Geometry check sheet. Reference: drawing and pictorial views, mm from the part's lowest x, y, z. Round coordinates to 2 decimals unless told otherwise and drop trailing zeros. Write each loop counter-clockwise with the first axis right and the second up, starting at its lowest first coordinate (ties: lowest second). Pieces come first, ordered by that corner, then holes. Notation, with made-up numbers: M 86,75.25 L 115,75.25 A29 cw 115,114.25 Z; hole C -8,85 d3. An arc over 180 degrees is marked long. One line per question, with ' | ' between items.
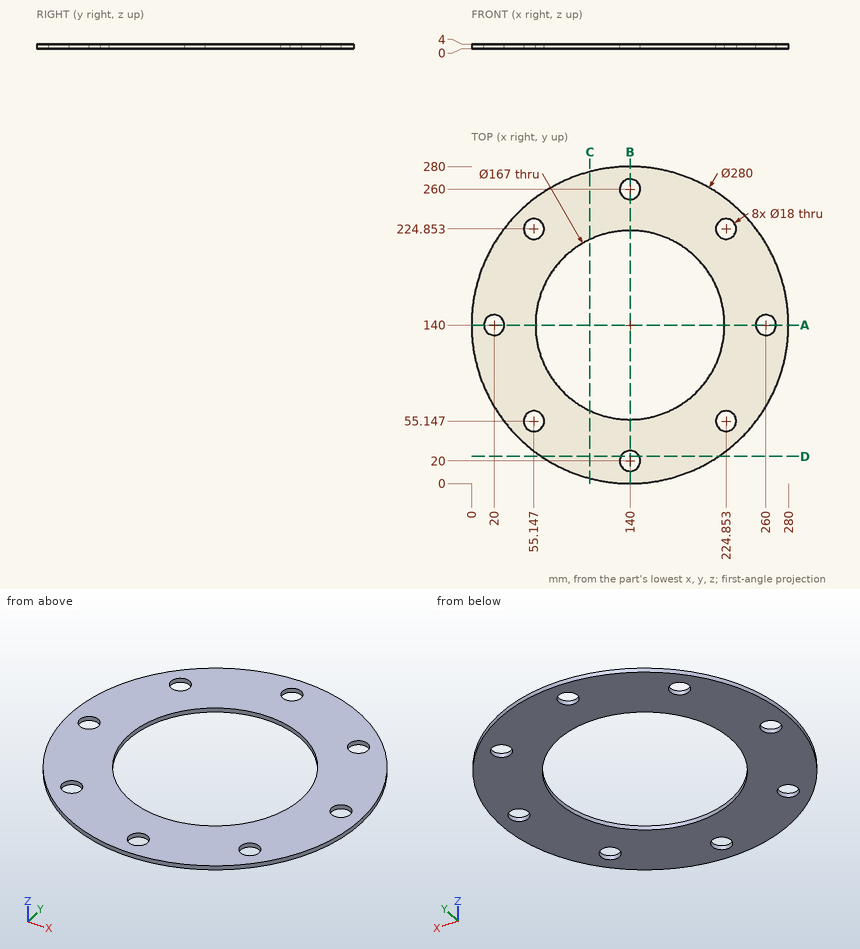
1. Go/stop test with flat-tipped pins: P1, Ø16, axis at x = 20, y = 140, coming from the +Z side; P2, Ø23.5, axis at x = 224.85, y = 55.15, coming from the -Z side; P3, Ø1.5, axis at y = 109.5, z = 3.5, coming from the -X side; P4, Ø1, axis at x = 133, z = 1.5, coming from the +Y side. Record where each tip stops, or that it passes through.
Results:
P1: passes through | P2: stops at z = 0 | P3: stops at x = 3.2 | P4: stops at y = 279.85
2. Thickness scan on line 1 (Y direction, x = 140, z = 1.9); line 2 (Y direction, x = 54, z = 1.35); line 3 (X direction, y = 135.5, z = 1.25) (1 decimal). Record the ranges inside material, lowest first.
Results:
line 1: y = 0 to 11, 29 to 56.5, 223.5 to 251, 269 to 280 | line 2: y = 29.53 to 46.22, 64.07 to 215.93, 233.78 to 250.47 | line 3: x = 0.1 to 12.2, 27.8 to 56.6, 223.4 to 252.2, 267.8 to 279.9
3. Section check D-D, the plane y = 24. Record the cut outline in (x, z).
Results:
outline: M 61.62,0 L 131.94,0 L 131.94,4 L 61.62,4 Z; M 148.06,0 L 218.38,0 L 218.38,4 L 148.06,4 Z
4. Section check C-C, the plane x = 104.5. Record the cut outline in (y, z).
Results:
outline: M 4.58,0 L 64.42,0 L 64.42,4 L 4.58,4 Z; M 215.58,0 L 275.42,0 L 275.42,4 L 215.58,4 Z
5. Section check A-A, the plane y = 140. Record the cut outline in (x, z).
Results:
outline: M 0,0 L 11,0 L 11,4 L 0,4 Z; M 29,0 L 56.5,0 L 56.5,4 L 29,4 Z; M 223.5,0 L 251,0 L 251,4 L 223.5,4 Z; M 269,0 L 280,0 L 280,4 L 269,4 Z
